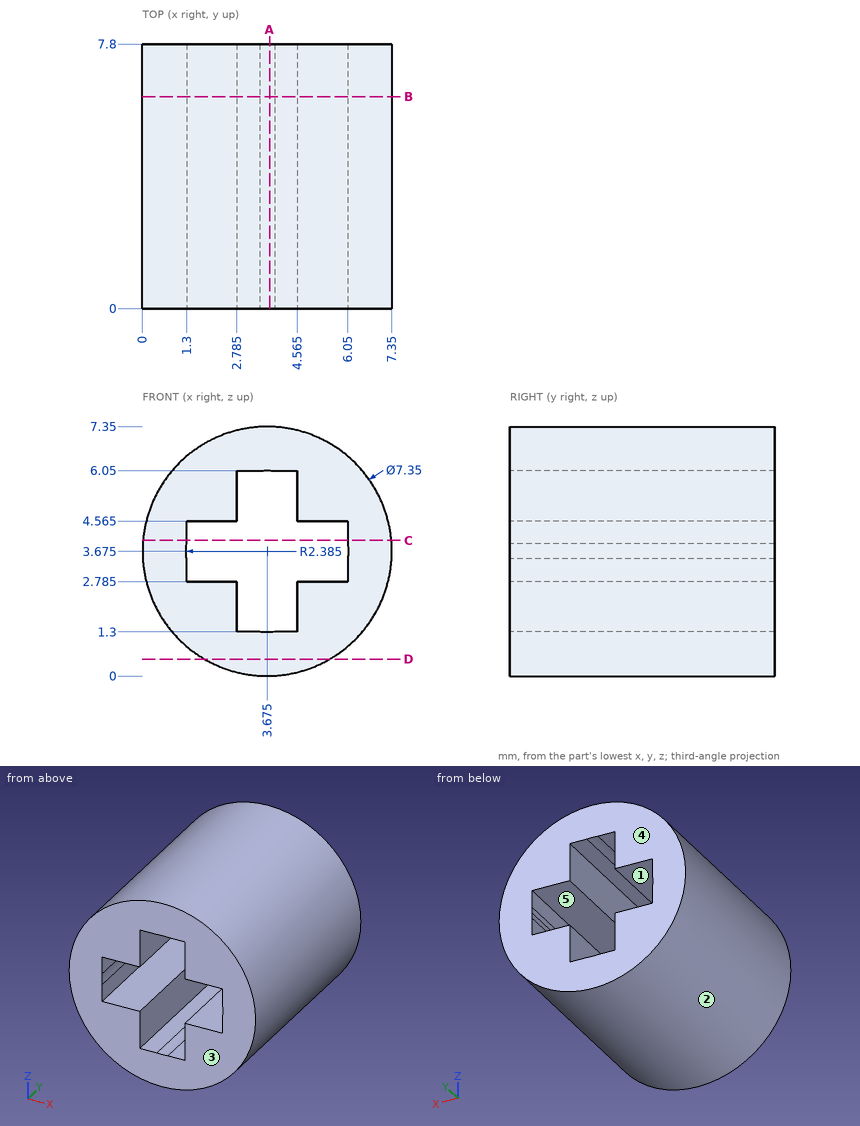
Could you check a few things on this drawing? It's one solid part, dimensions in mm from its lowest x, y, z. A direction names the side the tool comes from. Round coordinates to 2 decimals unless told otherwise and drop trailing zeros. Loops run counter-clockwise (first coordinate to the right, second up) from the corner with the lowest first, then second, coordinate; pieces in that order, holes last.
Q1. Thinking about a two-plate mould opening in X: for the marked faces 1, 2 and 3, which applies, pulls with the +X half, pulls with the -X half, needs draft (parallel to the pull), parting line crosses it, or undercut?
Q2. I want a section at B-B (y = 6.25). Write out the boundary of the cut face in (x, z) (3 decimals).
Q3. I want a section at D-D (z = 0.5). Write out the boundary of the cut face in (x, y), and give its area (3 significant figures).
Q4. Please list where these lines run through material, in increasing order: L1, parallel to X at y = 4.5, z = 3.75; L2, parallel to X at y = 2.25, z = 1.75 (1 decimal); L3, parallel to Z at x = 2, y = 6.75 (3 decimals).
Q5. For P1, Ø1.6, axis at x = 2, y = 3, coming from the +Z side; P2, Ø1.6, axis at x = 5, y = 5, coming from the +Z side; P3, Ø1.6, axis at y = 4, z = 2, coming from the +X side, each with a flat end and sliding along its axis, tell me the tip position at first contact or that it passes through.
Q6. I want a section at C-C (z = 4). Write out the boundary of the cut face in (x, y).
Q7. I want a section at A-A (x = 3.75). Write out the boundary of the cut face in (y, z), and give its area (3 significant figures).
Q8. On a 3-axis mill with a long thin cutter (end or side, diameter ignored), from which of +Z, -Z, +X, -X, +Y, -Y can I reach the whole of each face in a straight line? I mean the marked faces 4 and 5. Say none if no direction works.
Answer below:
1. face 1: undercut
1. face 2: parting line crosses it
1. face 3: needs draft
2. outline: circle Ø7.35 at (3.675, 3.675); hole (1.3, 2.785) - (2.785, 2.785) - (2.785, 1.3) - (3.457, 1.3) arc R2.385 ccw to (3.893, 1.3) - (4.565, 1.3) - (4.565, 2.785) - (6.05, 2.785) - (6.05, 3.457) arc R2.385 ccw to (6.05, 3.893) - (6.05, 4.565) - (4.565, 4.565) - (4.565, 6.05) - (3.893, 6.05) arc R2.385 ccw to (3.457, 6.05) - (2.785, 6.05) - (2.785, 4.565) - (1.3, 4.565) - (1.3, 3.893) arc R2.385 ccw to (1.3, 3.457) - close
3. outline: (1.82, 0) - (5.53, 0) - (5.53, 7.8) - (1.82, 7.8) - close
3. area: 28.9 mm2
4. L1: x = 0 to 1.29, 6.06 to 7.35
4. L2: x = 0.5 to 2.8, 4.6 to 6.8
4. L3: z = 0.404 to 2.785, 4.565 to 6.946
5. P1: stops at z = 7.24
5. P2: stops at z = 7.31
5. P3: stops at x = 7.24
6. outline: (0.01, 0) - (1.3, 0) - (1.3, 7.8) - (0.01, 7.8) - close; (6.05, 0) - (7.34, 0) - (7.34, 7.8) - (6.05, 7.8) - close
7. outline: (0, 0) - (7.8, 0) - (7.8, 1.29) - (0, 1.29) - close; (0, 6.06) - (7.8, 6.06) - (7.8, 7.35) - (0, 7.35) - close
7. area: 20.1 mm2
8. face 4: +Z, -Z, +X, -X, +Y
8. face 5: +Y, -Y
